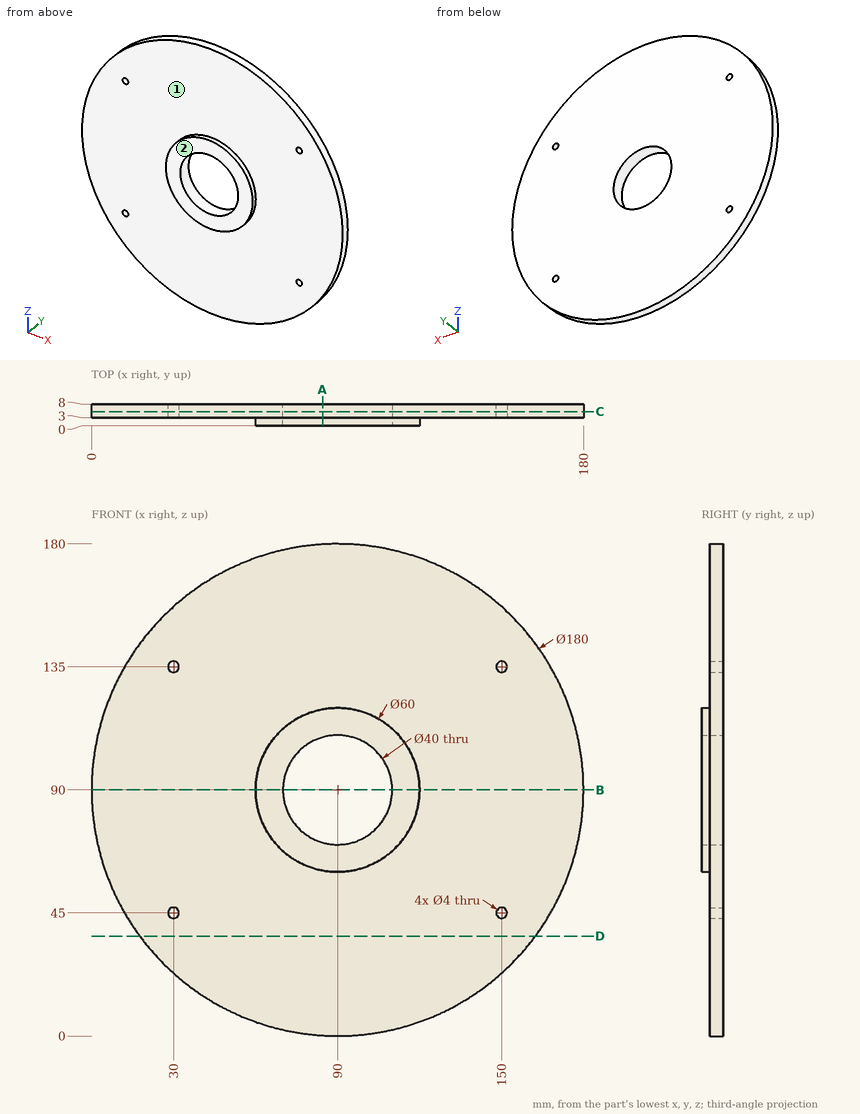
The drawing under review shows one solid part. Ordinate dimensions are in mm from its lowest x, y, z. A direction names the side the tool comes from. Give positions to 0.01 mm unless a question says otherwise; leave off trailing zeros. Loops run counter-clockwise (first coordinate to the right, second up) from the corner with the lowest first, then second, coordinate; pieces in that order, holes last. Notation, with made-up numbers: M -15.75,47 L -6.75,47 A16 ccw -6.75,61 Z; hole C 65.5,66.5 d5. An arc over 180 degrees is marked long. Return JSON: item names as keys, results as strings. Group by question number.
Item 1: We need section D-D (z = 36.5). Give the boundary of the cut face in (x, y), and give its area (3 significant figures).
Item 2: For probe 1 along Z at (x, y) = (90, 4.25); probe 2 along X at (y, z) = (7.25, 46.5); probe 3 along Z at (x, y) = (30, 4.85), list the stretches that pass through material, from the lowest coordinate up.
Item 3: Tool access review of the marked faces 1 and 2: name each direction out of +Z, -Z, +X, -X, +Y, -Y from which nothing blocks a thin tool from reaching the whole face with its end or side.
Item 4: Insertion check: pin 1 Ø5 at (x, z) = (150, 135) entering from -Y; pin 2 Ø2 at (x, y) = (32, 7) entering from -Z; pin 3 Ø4 at (x, y) = (22, 3.5) entering from -Z. Each pin has a flat end and moves straight along its axis. Give the tip position at first contact, or say it passes through.
Item 5: We need section B-B (z = 90). Give the boundary of the cut face in (x, y), and give its area (3 significant figures).
Item 6: We need section A-A (x = 84.5). Give the boundary of the cut face in (y, z), and give its area (3 significant figures).
Item 7: We need section C-C (y = 5.25). Give the boundary of the cut face in (x, z), and give its area (3 significant figures).
Output:
{
 "1": {"outline": "M 17.63,3 L 162.37,3 L 162.37,8 L 17.63,8 Z", "area": "724 mm^2"},
 "2": {"probe 1": "z = 0 to 70, 110 to 180", "probe 2": "x = 11.21 to 28.68, 31.32 to 148.68, 151.32 to 168.79", "probe 3": "z = 22.92 to 43, 47 to 133, 137 to 157.08"},
 "3": {"face 1": "-Y", "face 2": "+Z, -Z, +X, -X, -Y"},
 "4": {"pin 1": "stops at y = 3", "pin 2": "stops at z = 20.35", "pin 3": "stops at z = 28.81"},
 "5": {"outline": "M 0,3 L 60,3 L 60,0 L 70,0 L 70,8 L 0,8 Z; M 110,0 L 120,0 L 120,3 L 180,3 L 180,8 L 110,8 Z", "area": "760 mm^2"},
 "6": {"outline": "M 0,60.51 L 3,60.51 L 3,0.17 L 8,0.17 L 8,70.77 L 0,70.77 Z; M 0,109.23 L 8,109.23 L 8,179.83 L 3,179.83 L 3,119.49 L 0,119.49 Z", "area": "768 mm^2"},
 "7": {"outline": "C 90,90 d180; hole C 30,45 d4; hole C 30,135 d4; hole C 90,90 d40; hole C 150,45 d4; hole C 150,135 d4", "area": "24,100 mm^2"}
}
